Can you work these out from the model? Positions are in its coordinate system, mm. A direction names the side the tool comes from. Round coordinates to 2 decimals unless told otherwise and drop trailing zeros. Write each loop counter-clockwise with the first axis right and the second up, starting at its lowest first coordinate (ties: lowest second). Pieces come first, ordered by that corner, then holes. Notation, with made-up numbers: M -38,-21 L 8,-21 A23 cw 8,-10 Z; hole C 24,2.5 d11. An arc over 180 degrees is marked long. Answer in a Markdown table with one row per item. Add a question column.
(1) Suppose I cut it at A-A, the plane x = -52. Write out the boundary of the cut face in (y, z), then the cut area to 3 significant figures.
(2) If I drill on probe 1 along Y at (x, z) = (-52, 3.5); probe 2 along X at (y, z) = (-7.5, 2.5); probe 3 along Y at (x, z) = (-13, 8), over which ranges is the centre line in solid material (lowest first)?
(3) I'm going to push flat-ended pins straight in: pin 1 (3.5 mm diameter, centred on x = -52, y = -7.5, fed in from +Z); pin 2 (3 mm diameter, centred on x = 52, y = -7.5, fed in from -Z). Where does each tip first touch, or does it pass through?
(4) For faces 4 (the face through (-1, 0, 3)), 5 (the face through (53, -4, 4)), 6 (the face through (-1, -1.5, 7)), which set-ups out of +Z, -Z, +X, -X, +Y, -Y let a thin tool reach every point of the face, with its end or its side?
(5) If we mould it in two halves opening along Z, with no side actions, what happens to faces 1 (the face through (-1, 3, 9)), 2 (the face through (-1, 1.5, 7)), 3 (the face through (1, -5, 4))? For each: released by +Z, released by -Z, zero draft, split by the parting line, or undercut.
(6) Suppose I cut it at B-B, the plane y = 7.5. Write out the boundary of the cut face in (x, z).
(7) Suppose I cut it at C-C, the plane x = -18. Write out the boundary of the cut face in (y, z), then the cut area to 3 significant figures.
from build123d import *

# Parameters (mm, degrees)
SKETCH_W              = 111
SKETCH_H              = 22
PAD_DEPTH             = 3
PAD001_DEPTH          = 3
SKETCH002_W           = 111
SKETCH002_H           = 22
SKETCH002_W_2         = 95.5
SKETCH002_H_2         = 3
PAD002_DEPTH          = 3
SKETCH003_R           = 1.55
POCKET_DEPTH          = 236.034037
POLARPATTERN_COUNT    = 2
POLARPATTERN001_COUNT = 2
POLARPATTERN002_COUNT = 2
FILLET_R              = 2


with BuildPart() as part:
    # Sketch → Pad (new body)
    with BuildSketch(Plane.XY):
        Rectangle(SKETCH_W, SKETCH_H)
    extrude(amount=PAD_DEPTH)

    # Sketch001 (on Face6 of Pad) → Pad001 (join)
    with BuildSketch(Plane.XY.offset(3)):
        Polygon((-55.5, 11), (55.5, 11), (55.5, 4), (50, 4), (50, 5), (-50, 5), (-50, 4), (-55.5, 4), align=None)
        Polygon((-55.5, -11), (55.5, -11), (55.5, -4), (50, -4), (50, -5), (-50, -5), (-50, -4), (-55.5, -4), align=None)
    extrude(amount=PAD001_DEPTH)

    # Sketch002 (on Face12 of Pad001) → Pad002 (join)
    with BuildSketch(Plane.XY.offset(6)):
        Rectangle(SKETCH002_W, SKETCH002_H)
        Rectangle(SKETCH002_W_2, SKETCH002_H_2, mode=Mode.SUBTRACT)
    extrude(amount=PAD002_DEPTH)

    # Sketch003 (on Face26 of Pad002) → Pocket (cut, through all)
    with BuildSketch(Plane.XY.offset(9)):
        with Locations((-52, 7.5)):
            Circle(SKETCH003_R)
    pocket = extrude(amount=-POCKET_DEPTH, mode=Mode.SUBTRACT)

    # PolarPattern: Pocket ×2 about axis
    polarpattern_axis = Axis((0, 0, 0), (0, 1, 0))
    for i in range(1, POLARPATTERN_COUNT):
        add(pocket.rotate(polarpattern_axis, i * 360 / POLARPATTERN_COUNT), mode=Mode.SUBTRACT)

    # PolarPattern001: Pocket ×2 about axis
    polarpattern001_axis = Axis((0, 0, 0), (1, 0, 0))
    for i in range(1, POLARPATTERN001_COUNT):
        add(pocket.rotate(polarpattern001_axis, i * 360 / POLARPATTERN001_COUNT), mode=Mode.SUBTRACT)

    # PolarPattern002: Pocket ×2 about axis
    polarpattern002_axis = Axis((0, 0, 9), (0, 0, 1))
    for i in range(1, POLARPATTERN002_COUNT):
        add(pocket.rotate(polarpattern002_axis, i * 360 / POLARPATTERN002_COUNT), mode=Mode.SUBTRACT)

    # Fillet
    fillet_edges = [part.edges().sort_by_distance(p)[0] for p in [
        (55.5, 11, 7.5),
        (55.5, 11, 4.5),
        (55.5, 11, 1.5),
        (55.5, -11, 7.5),
        (-55.5, 11, 7.5),
        (-55.5, -11, 7.5),
    ]]
    fillet(fillet_edges, radius=FILLET_R)


solid = part.part
Calculated:
| question | item | result |
|---|---|---|
| 1 | outline | M -11,0 L -9.05,0 L -9.05,9 L -11,9 Z; M -5.95,0 L 5.95,0 L 5.95,9 L -5.95,9 Z; M 9.05,0 L 11,0 L 11,9 L 9.05,9 Z; hole M -4,3 L 4,3 L 4,6 L -4,6 Z |
| 1 | area | 118 mm² |
| 2 | probe 1 | -11 to -9.05, -5.95 to -4, 4 to 5.95, 9.05 to 11 |
| 2 | probe 2 | -55.5 to -53.55, -50.45 to 50.45, 53.55 to 55.5 |
| 2 | probe 3 | -11 to -1.5, 1.5 to 11 |
| 3 | pin 1 | z = 9 |
| 3 | pin 2 | through |
| 4 | face 4 | none |
| 4 | face 5 | +X, -X |
| 4 | face 6 | +Z |
| 5 | face 1 | released by +Z |
| 5 | face 2 | zero draft |
| 5 | face 3 | undercut |
| 6 | outline | M -55.5,0 L -53.55,0 L -53.55,9 L -55.5,9 Z; M -50.45,0 L 50.45,0 L 50.45,9 L -50.45,9 Z; M 53.55,0 L 55.5,0 L 55.5,9 L 53.55,9 Z |
| 7 | outline | M -11,0 L 11,0 L 11,9 L 1.5,9 L 1.5,6 L 5,6 L 5,3 L -5,3 L -5,6 L -1.5,6 L -1.5,9 L -11,9 Z |
| 7 | area | 159 mm² |
